For this review, take the finished solid that the model builds, in its own axes (mm). Face numbers are marked on the shaded views. A direction names the side the tool comes from. Give positions to 0.01 mm unless a question says otherwise; leave off trailing zeros. Order: outer loops, then holes, each group sorted by start corner. A loop starts at its lowest first (then second) coordinate and runs counter-clockwise, first axis right, second up. Notation, with made-up numbers: M 56,71.25 L 99,71.25 A30 cw 99,98.25 Z; hole C -31,-30.5 d7. An arc over 180 degrees is marked long. Answer as CSV lines item,"result". Start each with the question number.
1. Machinability: for the marked faces 1 and 2, which of the approach directions +Z, -Z, +X, -X, +Y, -Y give a long, thin tool a straight path to every point of the face, cutting with its end or side? Answer none if there is none.
2. We need section C-C, the plane x = 4.5. Give the boundary of the cut face in (y, z).
3. For line 1 along X through (y, z) = (-0.1, 1.3); line 2 along X through (y, z) = (1.9, 0.45); line 3 along Z through (x, y) = (16.5, 1), list the stretches that pass through material, from the lowest coordinate up.
4. We need section D-D, the plane x = 33. Give the boundary of the cut face in (y, z).
5. Clearance check with flat-ended pins moving along their axes: P1, Ø1, axis at x = 6, y = -1.5, coming from the +Z side; P2, Ø2, axis at x = 20, y = -1.5, coming from the -Z side; P3, Ø1.2, axis at y = -1, z = 1, coming from the -X side. State where each tip first meets the part, or that it passes through.
6. We need section A-A, the plane y = 0. Give the boundary of the cut face in (x, z), and give its area (3 significant figures).
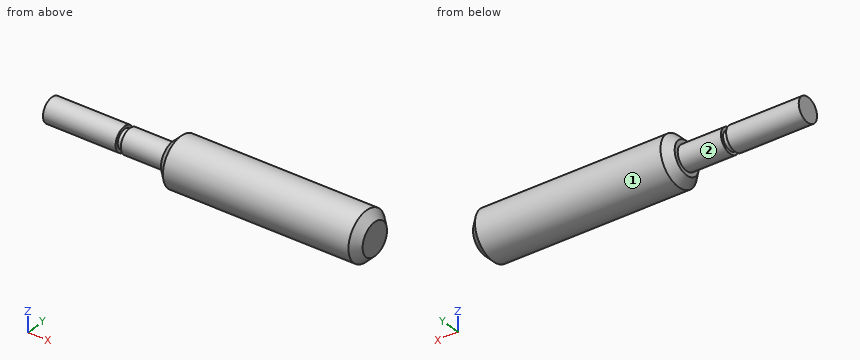
Autodesk Inventor part; units mm, degrees
ref_plane "YZ Plane" through (0, 0, 0) normal (1, 0, 0) x (0, 1, 0)
ref_plane "XZ Plane" through (0, 0, 0) normal (0, 1, 0) x (-1, 0, 0)
ref_plane "XY Plane" through (0, 0, 0) normal (0, 0, 1) x (1, 0, 0)
sketch "Skizze1" plane through (0, 0, 0) normal (0, 0, 1) x (1, 0, 0)
  line L0 (-8, 0) -> (48, 0)
  line L1 (0, -0.6) -> (0, 3.6)
  line L2 (0, 1.5) -> (9, 1.5)
  line L3 (9, 1.15) -> (9.64, 1.15)
  line L4 (9.64, 1.15) -> (9.64, 1.5)
  line L5 (9.64, 1.5) -> (15, 1.5)
  line L6 (15, 1.5) -> (15, 3)
  line L7 (15, 3) -> (40, 3)
  line L8 (40, 3) -> (40, 0)
  line L9 (40, 0) -> (0, 0)
  line L10 (0, 0) -> (0, 1.5)
  line L11 (9, 1.5) -> (9, 1.15)
  dimension "d0" = 3
  dimension "d1" = 2.3
  dimension "d2" = 9
  dimension "d3" = 0.64
  dimension "d4" = 3
  dimension "d5" = 15
  dimension "d6" = 40
  dimension "d7" = 6
revolve "Umdrehung1" add sketch "Skizze1" angle 360 about axis through (-10, 0, 0) along (1, 0, 0)
thread "Gewinde2"
chamfer "Fase1" distance 1 angle 45 2 edges at (15, -3, 0) (40, -3, 0)
properties part number "13_1087_035"
Result set:
1,face 1,"+X, -X"
1,face 2,"-X"
2,outline,"C 0,0 d3"
3,line 1,"0 to 9, 9.64 to 40"
3,line 2,"15 to 40"
3,line 3,"-2.83 to 2.83"
4,outline,"C 0,0 d6"
5,P1,"z = 1.12"
5,P2,"z = -2.96"
5,P3,"x = 0"
6,outline,"M 0,-1.5 L 9,-1.5 L 9,-1.15 L 9.64,-1.15 L 9.64,-1.5 L 15,-1.5 L 15,-2 L 16,-3 L 39,-3 L 40,-2 L 40,2 L 39,3 L 16,3 L 15,2 L 15,1.5 L 9.64,1.5 L 9.64,1.15 L 9,1.15 L 9,1.5 L 0,1.5 Z"
6,area,"193 mm2"
